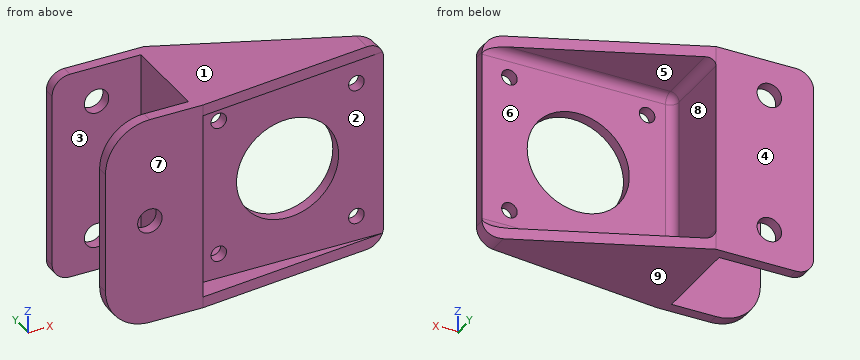
Autodesk Inventor part; units mm, degrees
ref_plane "YZ Plane" through (0, 0, 0) normal (1, 0, 0) x (0, 1, 0)
ref_plane "XZ Plane" through (0, 0, 0) normal (0, 1, 0) x (-1, 0, 0)
ref_plane "XY Plane" through (0, 0, 0) normal (0, 0, 1) x (1, 0, 0)
sketch "Sketch1" plane through (0, 0, 0) normal (0, 0, 1) x (1, 0, 0)
  line L0 (0, 0) -> (20, 0)
  line L1 (20, 0) -> (20, 2.5) construction
  line L2 (20, 2.5) -> (0, 2.5)
  line L3 (0, 2.5) -> (0, 0)
  line L4 (0, 25.3) -> (20, 25.3)
  line L5 (20, 25.3) -> (20, 22.8) construction
  line L6 (20, 22.8) -> (0, 22.8)
  line L7 (0, 22.8) -> (0, 25.3)
  line L8 (20, 22.8) -> (20, 2.5)
  line L9 (20, 25.3) -> (22, 25.3)
  line L10 (22, 25.3) -> (65.3, 7.5) construction
  line L11 (65.3, 7.5) -> (65.3, 5)
  line L12 (65.3, 5) -> (22, 0) construction
  line L13 (22, 0) -> (20, 0)
  line L14 (22, 25.3) -> (22, 0) construction
  line L15 (22, 25.3) -> (22, 7.5)
  line L16 (65.3, 7.5) -> (22, 7.5)
  line L17 (65.3, 5) -> (22, 5)
  line L18 (22, 5) -> (22, 0)
  dimension "d0" = 2.5
  dimension "d1" = 2.5
  dimension "d2" = 20
  dimension "d3" = 20.3
  dimension "d4" = 2
  dimension "d5" = 43.3
  dimension "d6" = 5
  dimension "d7" = 2.5
extrude "Extrusion1" add sketch "Sketch1" along normal mid plane 42.3
sketch "Sketch2" plane through (0, 0, 21.15) normal (0, 0, 1) x (1, 0, 0)
  line L0 (65.3, 5) -> (65.3, 7.5)
  line L1 (65.3, 7.5) -> (22, 7.5) construction
  line L2 (22, 7.5) -> (22, 25.3) construction
  line L3 (22, 25.3) -> (0, 25.3)
  line L4 (0, 25.3) -> (0, 22.8)
  line L5 (0, 22.8) -> (20, 22.8)
  line L6 (20, 22.8) -> (20, 2.5)
  line L7 (20, 2.5) -> (0, 2.5)
  line L8 (0, 2.5) -> (0, 0)
  line L9 (0, 0) -> (22, 0)
  line L10 (22, 0) -> (22, 5) construction
  line L11 (22, 5) -> (65.3, 5) construction
  line L12 (22, 7.5) -> (22, 25.3) construction
  line L13 (22, 25.3) -> (65.3, 7.5)
  line L14 (65.3, 5) -> (65.3, 7.5)
  line L15 (65.3, 5) -> (22, 0)
extrude "Extrusion2" add sketch "Sketch2" along normal blind 2.5
mirror "Mirror1" about plane through (0, 0, 0) normal (0, 0, 1) of "Extrusion2"
sketch "Sketch3" plane through (0, 25.3, 23.65) normal (0, 1, 0) x (1, 0, 0)
  line L0 (0, 47.3) -> (22, 47.3)
  line L1 (10, 47.3) -> (10, 0) construction
  line L2 (0, 0) -> (20, 0)
  circle A0 centre (10, 8) radius 2.75
  circle A1 centre (10, 39.3) radius 2.75
  line L3 (0, 47.3) -> (0, 0)
  point P0 (0, 23.65)
  dimension "d12" = 8
  dimension "d13" = 8
  dimension "d14" = 5.5
  dimension "d15" = 10
extrude "Extrusion3" cut sketch "Sketch3" against normal up to surface (2.5 mm away)
sketch "Sketch4" plane through (0, 0, 23.65) normal (0, -1, 0) x (1, 0, 0)
  line L0 (0, -23.65) -> (10, -23.65) construction
  circle A0 centre (10, -23.65) radius 2.75
  dimension "d18" = 5.5
  dimension "d19" = 10
extrude "Extrusion4" cut sketch "Sketch4" against normal up to surface (2.5 mm away)
sketch "Sketch5" plane through (22, 7.5, 21.15) normal (0, 1, 0) x (1, 0, 0)
  line L0 (0, 0) -> (0, -2.5)
  line L1 (43.3, 42.3) -> (43.3, 44.8)
  line L2 (0, 0) -> (43.3, 42.3) construction
  line L3 (6.15, 5.65) -> (37.15, 5.65) construction
  line L4 (37.15, 5.65) -> (37.15, 36.65) construction
  line L5 (37.15, 36.65) -> (6.15, 36.65) construction
  line L6 (6.15, 36.65) -> (6.15, 5.65) construction
  line L7 (6.15, 5.65) -> (37.15, 36.65) construction
  line L8 (37.15, 5.65) -> (6.15, 36.65) construction
  circle A0 centre (6.15, 36.65) radius 1.75
  circle A1 centre (37.15, 36.65) radius 1.75
  circle A2 centre (37.15, 5.65) radius 1.75
  circle A3 centre (6.15, 5.65) radius 1.75
  circle A4 centre (21.65, 21.15) radius 11.5
  point P0 (-22, 21.15)
  dimension "d22" = 31
  dimension "d23" = 31
  dimension "d24" = 3.5
  dimension "d25" = 23
extrude "Extrusion5" cut sketch "Sketch5" against normal through all
fillet "Fillet1" radius 10 2 edges at (0, 1.25, -23.65) (0, 1.25, 23.65)
fillet "Fillet1" radius 4 4 edges at (0, 24.05, -23.65) (0, 24.05, 23.65) (65.3, 6.25, 23.65) (65.3, 6.25, -23.65)
fillet "Fillet1" radius 2 5 edges at (43.65, 7.5, -21.15) (22, 7.5, 0) (43.65, 7.5, 21.15) (22, 16.4, 21.15) (22, 16.4, -21.15)
properties part number "MotorBracket2"
Geometry: final body of the model. Coordinates: model frame, mm. Face numbers are marked on the shaded views. A direction names the side the tool comes from. Give positions to 0.01 mm unless a question says otherwise; leave off trailing zeros. Write each loop counter-clockwise with the first axis right and the second up, starting at its lowest first coordinate (ties: lowest second). Pieces come first, ordered by that corner, then holes.
1. Reachability of the marked faces 1, 2, 3, 4 and 5 from +Z, -Z, +X, -X, +Y, -Y: full face, straight path, thin tool, end or side. Return the list, or none.
2. Section query A-A, the plane x = 15. Return loops of the section in (y, z).
3. Pin query (flat end, axial travel): P1, Ø4, axis at y = 2.5, z = -1, coming from the +X side; P2, Ø10, axis at y = 9, z = 2.5, coming from the -X side; P3, Ø5, axis at x = 29, z = 15, coming from the +Y side. Return the tip coordinate at first contact, or that it passes through.
4. Section query B-B, the plane z = -8.5. Return loops of the section in (x, y), then the cut area to 3 significant figures.
5. Line query: probe 1 along X at (y, z) = (6.9, -15.5); probe 2 along Y at (x, z) = (18.5, 6.5); probe 3 along Z at (x, y) = (43.65, 5.7). Output: solid intervals per line, ascending.
6. Section query C-C, the plane x = 59.15. Return loops of the section in (y, z), then the cut area to 3 significant figures.
7. Draft query along Z for the marked faces 6, 7, 8 and 9. Return one class per face: released by +Z, released by -Z, zero draft, split by the parting line, or undercut.
8. Section query D-D, the plane z = 1.5. Return loops of the section in (x, y).
Computed:
1. face 1: +Z, +X, -X, +Y, -Y
1. face 2: +X, -Y
1. face 3: +Z, -Z, -X
1. face 4: +Z, -Z, +X, -X, +Y
1. face 5: +X, +Y
2. outline: (0, -23.65) - (2.5, -23.65) - (2.5, 23.65) - (0, 23.65) - close; (22.8, -23.65) - (25.3, -23.65) - (25.3, 23.65) - (22.8, 23.65) - close
3. P1: stops at x = 22
3. P2: stops at x = 20
3. P3: stops at y = 7.5
4. outline: (0, 0) - (22, 0) - (22, 5) - (35.9, 5) - (35.9, 7.5) - (24, 7.5) arc R2 cw to (22, 9.5) - (22, 25.3) - (0, 25.3) - (0, 22.8) - (20, 22.8) - (20, 2.5) - (0, 2.5) - close; (51.4, 5) - (65.3, 5) - (65.3, 7.5) - (51.4, 7.5) - close
4. area: 221 mm2
5. probe 1: x = 20 to 26.4, 29.9 to 57.4, 60.9 to 65.3
5. probe 2: y = 0 to 2.5, 22.8 to 25.3
5. probe 3: z = -23.65 to -11.5, 11.5 to 23.65
6. outline: (4.29, -23.65) - (10.03, -23.65) - (10.03, -21.15) - (9.5, -21.15) arc R2 cw to (7.5, -19.15) - (7.5, -17.25) - (5, -17.25) - (5, -21.15) - (4.29, -21.15) - close; (4.29, 21.15) - (5, 21.15) - (5, 17.25) - (7.5, 17.25) - (7.5, 19.15) arc R2 cw to (9.5, 21.15) - (10.03, 21.15) - (10.03, 23.65) - (4.29, 23.65) - close; (5, -13.75) - (7.5, -13.75) - (7.5, 13.75) - (5, 13.75) - close
6. area: 119 mm2
7. face 6: undercut
7. face 7: zero draft
7. face 8: undercut
7. face 9: released by -Z
8. outline: (0, 0) - (7.7, 0) - (7.7, 2.5) - (0, 2.5) - close; (0, 22.8) - (20, 22.8) - (20, 2.5) - (12.3, 2.5) - (12.3, 0) - (22, 0) - (22, 5) - (32.25, 5) - (32.25, 7.5) - (24, 7.5) arc R2 cw to (22, 9.5) - (22, 25.3) - (0, 25.3) - close; (55.05, 5) - (65.3, 5) - (65.3, 7.5) - (55.05, 7.5) - close
